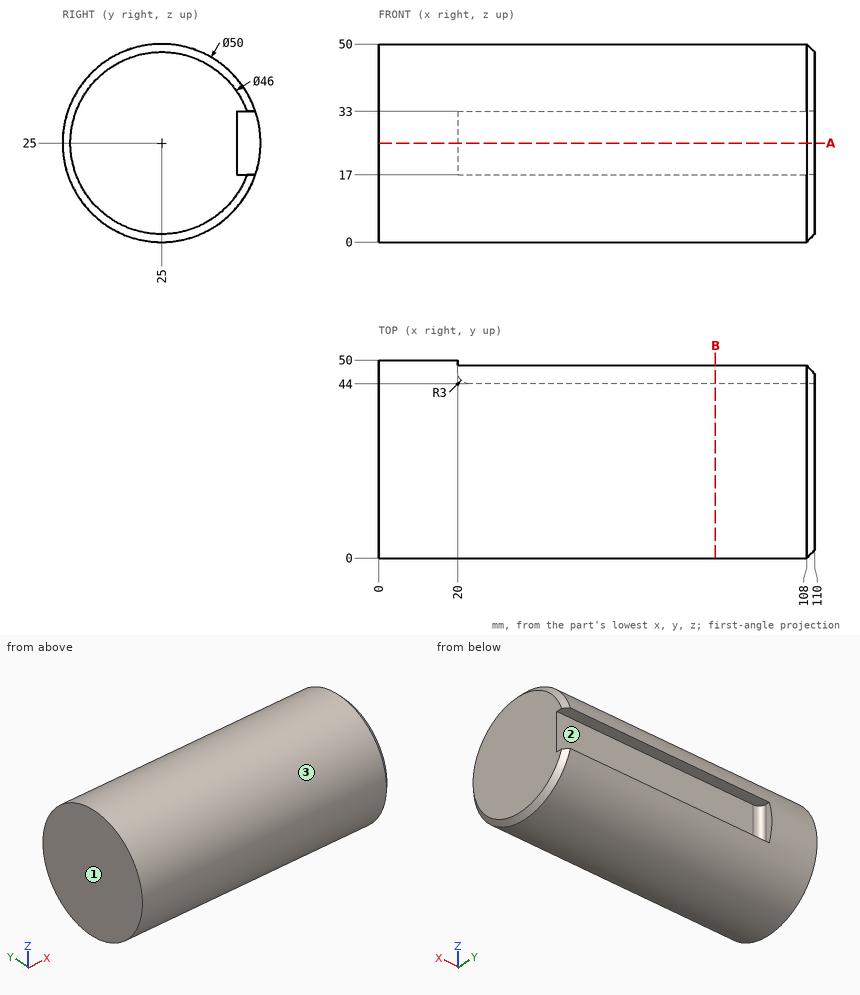
Could you check a few things on this drawing? It's one solid part, dimensions in mm from its lowest x, y, z. Coordinates: 2 decimals unless noted, no trailing zeros. Order: outer loops, then holes, each group sorted by start corner. A loop starts at its lowest first (then second) coordinate and runs counter-clockwise, first axis right, second up. Notation, with made-up numbers: (9.5, 85.5) - (49.5, 85.5) arc R11 cw to (49.5, 100.5) - close; hole circle Ø2 at (-23, 50.5). An arc over 180 degrees is marked (long way). One line per question, with ' | ' between items. Start each with the question number.
1. I'm going to push flat-ended pins straight in: pin 1 Ø8 at (x, z) = (64.5, 28) entering from +Y; pin 2 Ø6 at (x, y) = (83.5, 37.5) entering from -Z; pin 3 Ø2 at (x, y) = (91, 23) entering from +Z. Where does each tip first touch, or does it pass through?
2. If we mould it in two halves opening along Z, with no side actions, what happens to the marked faces 1, 2 and 3? For each: released by +Z, released by -Z, zero draft, split by the parting line, or undercut.
3. Please list where these lines run through material, in increasing order: line 1 along Z through (x, y) = (24.5, 46.5); line 2 along Z through (x, y) = (25, 7); line 3 along Y through (x, z) = (72, 46.5). Write a range as [from, to].
4. If we section it at B-B (x = 85): Write out the boundary of the cut face in (y, z).
5. If we section it at A-A (z = 25): Write out the boundary of the cut face in (x, y), and give its area (3 significant figures).
Model answer:
1) pin 1: stops at y = 44 | pin 2: stops at z = 1.88 | pin 3: stops at z = 49.98
2) face 1: zero draft | face 2: undercut | face 3: split by the parting line
3) line 1: z = [12.24, 17], [33, 37.76] | line 2: z = [7.65, 42.35] | line 3: y = [12.24, 37.76]
4) outline: (44, 17) - (44, 33) - (48.69, 33) arc R25 ccw (long way) to (48.69, 17) - close
5) outline: (0, 0) - (108, 0) - (110, 2) - (110, 44) - (23, 44) arc R3 cw to (20, 47) - (20, 50) - (0, 50) - close | area: 4,960 mm²
